Source: CAD feature listing. Evaluate the final solid. Frame: model axes, mm. Round coordinates to 2 decimals unless told otherwise and drop trailing zeros. Loops run counter-clockwise (first coordinate to the right, second up) from the corner with the lowest first, then second, coordinate; pieces in that order, holes last. Notation, with made-up numbers: (-38.75, 20) - (12.25, 20) arc R14 cw to (12.25, 40) - close; hole circle Ø7 at (69, 16). An arc over 180 degrees is marked (long way). Write item = value, one per line. Start each with the question number.
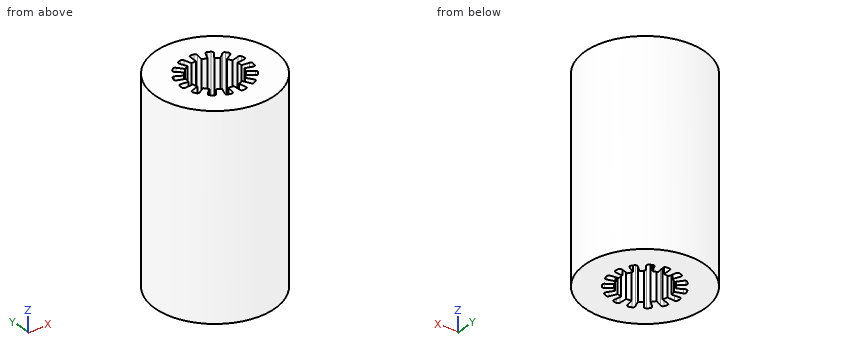
from build123d import *

# Parameters (mm, degrees)
F0_R     = 6
F1_DEPTH = 20


with BuildPart() as f1:
    # F0 (on Top) → F1 (new body)
    with BuildSketch(Plane.XY):
        Circle(F0_R)
        with BuildLine():
            Line((3.279786, 0.349242), (2.50894, 0.25))
            Line((2.50894, 0.25), (2.50894, -0.25))
            Line((2.50894, -0.25), (3.279786, -0.349242))
            ThreePointArc((3.279786, -0.349242), (3.414903, -0.428484), (3.451475, -0.580793))
            ThreePointArc((3.451475, -0.580793), (3.423517, -0.727691), (3.389309, -0.87326))
            ThreePointArc((3.389309, -0.87326), (3.293949, -0.997527), (3.138283, -1.01496))
            Line((3.138283, -1.01496), (2.393715, -0.792091))
            Line((2.393715, -0.792091), (2.190347, -1.248864))
            Line((2.190347, -1.248864), (2.854184, -1.653058))
            ThreePointArc((2.854184, -1.653058), (2.945389, -1.780405), (2.916849, -1.934423))
            ThreePointArc((2.916849, -1.934423), (2.831559, -2.057248), (2.741101, -2.176319))
            ThreePointArc((2.741101, -2.176319), (2.603441, -2.251056), (2.454143, -2.203667))
            Line((2.454143, -2.203667), (1.864595, -1.697223))
            Line((1.864595, -1.697223), (1.493022, -2.031788))
            Line((1.493022, -2.031788), (1.935067, -2.671045))
            ThreePointArc((1.935067, -2.671045), (1.966591, -2.824479), (1.877874, -2.953572))
            ThreePointArc((1.877874, -2.953572), (1.75, -3.031089), (1.618932, -3.103073))
            ThreePointArc((1.618932, -3.103073), (1.462775, -3.115357), (1.345659, -3.01134))
            Line((1.345659, -3.01134), (1.013069, -2.308889))
            Line((1.013069, -2.308889), (0.537541, -2.463398))
            Line((0.537541, -2.463398), (0.68136, -3.227184))
            ThreePointArc((0.68136, -3.227184), (0.647751, -3.380174), (0.514197, -3.462023))
            ThreePointArc((0.514197, -3.462023), (0.36585, -3.480827), (0.216834, -3.493277))
            ThreePointArc((0.216834, -3.493277), (0.069182, -3.440984), (0.004498, -3.298325))
            Line((0.004498, -3.298325), (-0.013625, -2.521328))
            Line((-0.013625, -2.521328), (-0.510886, -2.469064))
            Line((-0.510886, -2.469064), (-0.69016, -3.225313))
            ThreePointArc((-0.69016, -3.225313), (-0.783091, -3.351407), (-0.938389, -3.371858))
            ThreePointArc((-0.938389, -3.371858), (-1.081559, -3.328698), (-1.222756, -3.279462))
            ThreePointArc((-1.222756, -3.279462), (-1.336374, -3.171634), (-1.33744, -3.014999))
            Line((-1.33744, -3.014999), (-1.037964, -2.297806))
            Line((-1.037964, -2.297806), (-1.470976, -2.047806))
            Line((-1.470976, -2.047806), (-1.942346, -2.665757))
            ThreePointArc((-1.942346, -2.665757), (-2.078529, -2.743151), (-2.228719, -2.698668))
            ThreePointArc((-2.228719, -2.698668), (-2.341957, -2.601007), (-2.45092, -2.498598))
            ThreePointArc((-2.45092, -2.498598), (-2.510858, -2.35388), (-2.448123, -2.210353))
            Line((-2.448123, -2.210353), (-1.882829, -1.676972))
            Line((-1.882829, -1.676972), (-2.176721, -1.272464))
            Line((-2.176721, -1.272464), (-2.858682, -1.645267))
            ThreePointArc((-2.858682, -1.645267), (-3.014571, -1.660579), (-3.133684, -1.558854))
            ThreePointArc((-3.133684, -1.558854), (-3.197409, -1.423578), (-3.255298, -1.285704))
            ThreePointArc((-3.255298, -1.285704), (-3.251192, -1.129119), (-3.135503, -1.023516))
            Line((-3.135503, -1.023516), (-2.402136, -0.766175))
            Line((-2.402136, -0.766175), (-2.506092, -0.277101))
            Line((-2.506092, -0.277101), (-3.280726, -0.340295))
            ThreePointArc((-3.280726, -0.340295), (-3.429366, -0.290878), (-3.496806, -0.1495))
            ThreePointArc((-3.496806, -0.1495), (-3.5, 0), (-3.496806, 0.1495))
            ThreePointArc((-3.496806, 0.1495), (-3.429366, 0.290878), (-3.280726, 0.340295))
            Line((-3.280726, 0.340295), (-2.506092, 0.277101))
            Line((-2.506092, 0.277101), (-2.402136, 0.766175))
            Line((-2.402136, 0.766175), (-3.135503, 1.023516))
            ThreePointArc((-3.135503, 1.023516), (-3.251192, 1.129119), (-3.255298, 1.285704))
            ThreePointArc((-3.255298, 1.285704), (-3.197409, 1.423578), (-3.133684, 1.558854))
            ThreePointArc((-3.133684, 1.558854), (-3.014571, 1.660579), (-2.858682, 1.645267))
            Line((-2.858682, 1.645267), (-2.176721, 1.272464))
            Line((-2.176721, 1.272464), (-1.882829, 1.676972))
            Line((-1.882829, 1.676972), (-2.448123, 2.210353))
            ThreePointArc((-2.448123, 2.210353), (-2.510858, 2.35388), (-2.45092, 2.498598))
            ThreePointArc((-2.45092, 2.498598), (-2.341957, 2.601007), (-2.228719, 2.698668))
            ThreePointArc((-2.228719, 2.698668), (-2.078529, 2.743151), (-1.942346, 2.665757))
            Line((-1.942346, 2.665757), (-1.470976, 2.047806))
            Line((-1.470976, 2.047806), (-1.037964, 2.297806))
            Line((-1.037964, 2.297806), (-1.33744, 3.014999))
            ThreePointArc((-1.33744, 3.014999), (-1.336374, 3.171634), (-1.222756, 3.279462))
            ThreePointArc((-1.222756, 3.279462), (-1.081559, 3.328698), (-0.938389, 3.371858))
            ThreePointArc((-0.938389, 3.371858), (-0.783091, 3.351407), (-0.69016, 3.225313))
            Line((-0.69016, 3.225313), (-0.510886, 2.469064))
            Line((-0.510886, 2.469064), (-0.013625, 2.521328))
            Line((-0.013625, 2.521328), (0.004498, 3.298325))
            ThreePointArc((0.004498, 3.298325), (0.069182, 3.440984), (0.216834, 3.493277))
            ThreePointArc((0.216834, 3.493277), (0.36585, 3.480827), (0.514197, 3.462023))
            ThreePointArc((0.514197, 3.462023), (0.647751, 3.380174), (0.68136, 3.227184))
            Line((0.68136, 3.227184), (0.537541, 2.463398))
            Line((0.537541, 2.463398), (1.013069, 2.308889))
            Line((1.013069, 2.308889), (1.345659, 3.01134))
            ThreePointArc((1.345659, 3.01134), (1.462775, 3.115357), (1.618932, 3.103073))
            ThreePointArc((1.618932, 3.103073), (1.75, 3.031089), (1.877874, 2.953572))
            ThreePointArc((1.877874, 2.953572), (1.966591, 2.824479), (1.935067, 2.671045))
            Line((1.935067, 2.671045), (1.493022, 2.031788))
            Line((1.493022, 2.031788), (1.864595, 1.697223))
            Line((1.864595, 1.697223), (2.454143, 2.203667))
            ThreePointArc((2.454143, 2.203667), (2.603441, 2.251056), (2.741101, 2.176319))
            ThreePointArc((2.741101, 2.176319), (2.831559, 2.057248), (2.916849, 1.934423))
            ThreePointArc((2.916849, 1.934423), (2.945389, 1.780405), (2.854184, 1.653058))
            Line((2.854184, 1.653058), (2.190347, 1.248864))
            Line((2.190347, 1.248864), (2.393715, 0.792091))
            Line((2.393715, 0.792091), (3.138283, 1.01496))
            ThreePointArc((3.138283, 1.01496), (3.293949, 0.997527), (3.389309, 0.87326))
            ThreePointArc((3.389309, 0.87326), (3.423517, 0.727691), (3.451475, 0.580793))
            ThreePointArc((3.451475, 0.580793), (3.414903, 0.428484), (3.279786, 0.349242))
        make_face(mode=Mode.SUBTRACT)
    extrude(amount=F1_DEPTH)


solid = f1.part
(1) Cut plane A-A (y = -4.25). Output: boundary loops of the cut face in (x, z).
(2) Material intervals for line 1 along Y through (x, z) = (0.5, 5); line 2 along Y through (x, z) = (-5.5, 4.5); line 3 along X through (y, z) = (0.5, 9.75), sorted ascending. Write a range as from..to.
(3) Cut plane B-B (x = -4.5). Output: boundary loops of the cut face in (y, z).
(4) Pin query (flat end, axial travel): P1, Ø1, axis at y = -3.5, z = 13, coming from the +X side; P2, Ø1, axis at y = 3.5, z = 17.5, coming from the -X side; P3, Ø2, axis at x = 4, z = 3.5, coming from the +Y side. Return the tip coordinate at first contact, or that it passes through.
Solution:
q1.outline = (-4.24, 0) - (4.24, 0) - (4.24, 20) - (-4.24, 20) - close
q2.line_1 = -5.98..-3.46, 3.46..5.98
q2.line_2 = -2.4..2.4
q2.line_3 = -5.98..-2.46, 3.45..5.98
q3.outline = (-3.97, 0) - (3.97, 0) - (3.97, 20) - (-3.97, 20) - close
q4.P1 = 5.2
q4.P2 = -5.2
q4.P3 = 5.2
